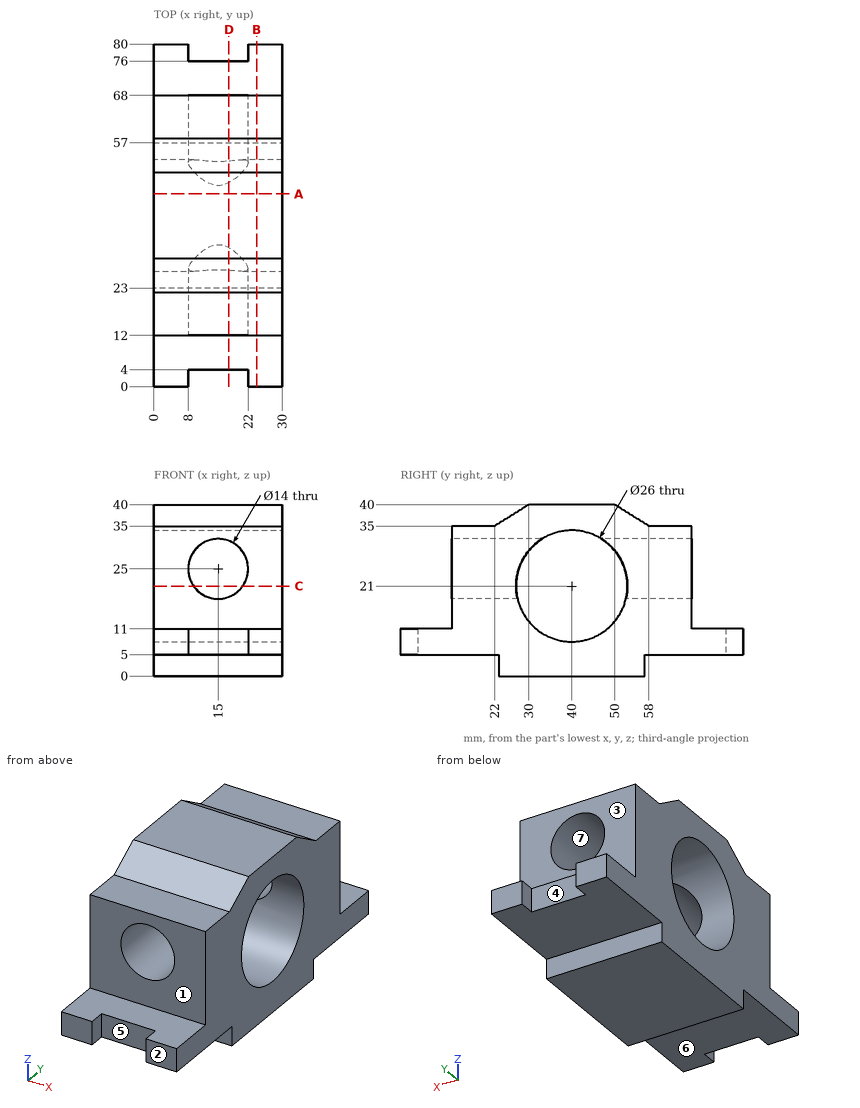
Answer from the drawing. Dimensions are ordinates in mm from the lowest x, y and z of the part. A direction names the side the tool comes from. Give positions to 0.01 mm unless a question says otherwise; leave off trailing zeros. Order: outer loops, then holes, each group sorted by start corner. A loop starts at its lowest first (then second) coordinate and runs counter-clockwise, first axis right, second up. Notation, with made-up numbers: (-16.5, 87.5) - (35.5, 87.5) arc R12 cw to (35.5, 105.5) - close; hole circle Ø6 at (36, 52). An arc over 180 degrees is marked (long way). One line per item, written item: value. Start each with the question number.
1) Find the intervals of material crossed by L1, parallel to Z at x = 15, y = 21.25; L2, parallel to X at y = 20, z = 25; L3, parallel to Y at x = 23.5, z = 10, in increasing order.
2) A tool of negligible diameter and unlimited length cuts with its end or side. For the marked faces 1, 2, 3 and 4, from which of +Z, -Z, +X, -X, +Y, -Y can it reach the whole face along a straight path? Write none if from no direction.
3) A cutting plane is placed at C-C on z = 21. Give the vertices of the cut face in (x, y).
4) A cutting plane is placed at A-A on y = 45. Give the vertices of the cut face in (x, z), then the cut area to 3 significant figures.
5) A cutting plane is placed at D-D on x = 17.5. Give the vertices of the cut face in (y, z), then the cut area to 3 significant figures.
6) The mould has two halves that part along Z. Classify the marked faces 5, 6 and 7: released by +Z, released by -Z, zero draft, split by the parting line, or undercut.
7) Given pin 1 Ø8.5 at (x, z) = (15, 25) entering from -Y; pin 2 Ø5 at (x, y) = (8.5, 63.5) entering from +Z; pin 3 Ø5 at (x, z) = (16, 8.5) entering from -Y; pin 4 Ø12 at (x, z) = (25.5, 20.5) entering from +Y, each flat-ended and moving along its own axis, determine where each tip first touches the part or whether it passes through.
8) A cutting plane is placed at B-B on x = 24. Give the vertices of the cut face in (y, z), then the cut area to 3 significant figures.
Answer sheet:
1. L1: z = 5 to 18, 32 to 35
1. L2: x = 0 to 8, 22 to 30
1. L3: y = 0 to 33.07, 46.93 to 80
2. face 1: +Z, +X, -X, -Y
2. face 2: +Z, -Z, +X, -X, -Y
2. face 3: +Z, +X, -X, +Y
2. face 4: +Z, -Z, +Y
3. outline: (0, 12) - (9.26, 12) - (9.26, 27) - (0, 27) - close; (0, 53) - (9.26, 53) - (9.26, 68) - (0, 68) - close; (20.74, 12) - (30, 12) - (30, 27) - (20.74, 27) - close; (20.74, 53) - (30, 53) - (30, 68) - (20.74, 68) - close
4. outline: (0, 0) - (30, 0) - (30, 9) - (0, 9) - close; (0, 33) - (30, 33) - (30, 40) - (0, 40) - close
4. area: 480 mm2
5. outline: (4, 5) - (23, 5) - (23, 0) - (57, 0) - (57, 5) - (76, 5) - (76, 11) - (68, 11) - (68, 18.46) - (52.75, 18.46) arc R13 cw to (27.25, 18.46) - (12, 18.46) - (12, 11) - (4, 11) - close; (12, 31.54) - (32.39, 31.54) arc R13 cw to (47.61, 31.54) - (68, 31.54) - (68, 35) - (58, 35) - (50, 40) - (30, 40) - (22, 35) - (12, 35) - close
5. area: 1,130 mm2
6. face 5: zero draft
6. face 6: released by -Z
6. face 7: undercut
7. pin 1: passes through
7. pin 2: stops at z = 35
7. pin 3: stops at y = 4
7. pin 4: stops at y = 68
8. outline: (0, 5) - (23, 5) - (23, 0) - (57, 0) - (57, 5) - (80, 5) - (80, 11) - (68, 11) - (68, 35) - (58, 35) - (50, 40) - (30, 40) - (22, 35) - (12, 35) - (12, 11) - (0, 11) - close; hole circle Ø26 at (40, 21)
8. area: 1,600 mm2
